Model file for the job. Use its own axes, mm. Give positions to 0.01 mm unless a question says otherwise; leave off trailing zeros. Loops run counter-clockwise (first coordinate to the right, second up) from the corner with the lowest first, then second, coordinate; pieces in that order, holes last. Notation, with made-up numbers: M -33.75,62 L 25.25,62 A17 cw 25.25,87 Z; hole C 69,12.5 d11. An arc over 180 degrees is marked long. Use CSV: the item, a comma, the result in double quotes. Start each with the question number.
(1) Wall check: line 1 along Y through (x, z) = (-37.05, 0.45); line 2 along Y through (x, z) = (-31.5, -0.8) (3 decimals); line 3 along Y through (x, z) = (27.05, -0.65). Give the ranges that are in metal, low to high. Write a range as from..to.
(2) Slice it at B-B on x = 27.05. List the corners of the cut face in (y, z).
(3) Slice it at C-C on y = -4.5. List the corners of the cut face in (x, z), and give its area (3 significant figures).
(4) Slice it at A-A on y = 12. List the corners of the cut face in (x, z) (3 decimals).
(5) Slice it at D-D on y = -19.5. List the corners of the cut face in (x, z).
(6) Flat gauge pins, fed straight in: P1, Ø0.9, axis at x = -25, z = -0.5, coming from the +Y side; P2, Ø4, axis at x = 31.5, y = 12, coming from the +Z side. Where does each tip first touch, or does it go through?
```python
from build123d import *

# Parameters (mm, degrees)
SKETCH_1_W                  = 93
SKETCH_1_H                  = 51
EXTRUDE_1_DEPTH             = 1.5
SKETCH_2_R                  = 1.525
CUT_EXTRUDE_1_DEPTH         = 5
HOLE_WIZARD_M3_1_AT_2_COUNT = 2
HOLE_WIZARD_M3_1_AT_2_PITCH = 63
SKETCH_5_R                  = 1.5
CUT_EXTRUDE_2_DEPTH         = 5
SKETCH_7_W                  = 20
SKETCH_7_H                  = 24
CUT_EXTRUDE_3_DEPTH         = 10
FILLET_1_R                  = 2
SKETCH_8_W                  = 16.1
SKETCH_8_H                  = 3.1
CUT_EXTRUDE_4_DEPTH         = 3
MIRROR_5_COPY_1_SKETCH_W    = 16.1
MIRROR_5_COPY_1_SKETCH_H    = 3.1
MIRROR_5_COPY_1_DEPTH       = 3
SKETCH_9_R                  = 1.025
CUT_EXTRUDE_5_DEPTH         = 3


with BuildPart() as part:
    # 草图1 → 凸台-拉伸1 (new body, symmetric)
    with BuildSketch(Plane.XY):
        Rectangle(SKETCH_1_W, SKETCH_1_H)
    extrude(amount=EXTRUDE_1_DEPTH, both=True)

    # 草图2 → 切除-拉伸1 (cut, symmetric)
    with BuildSketch(Plane.XY.offset(1.5)):
        with Locations((-31.5, 12)):
            Circle(SKETCH_2_R)
        with Locations((31.5, 12)):
            Circle(SKETCH_2_R)
    cut_extrude_1 = extrude(amount=CUT_EXTRUDE_1_DEPTH, both=True, mode=Mode.SUBTRACT)

    # 草图4 → M3 十字槽半沉头木螺钉的锥形沉头孔1 (revolve, cut)
    with BuildSketch(Plane(origin=(-31.5, 12, 1.5), x_dir=(0, -1, 0), z_dir=(1, 0, 0))):
        Polygon((0, 0), (0, 12.401290929), (1.5, 11.5), (1.5, 1.8), (3.3, 0), align=None)
    hole_wizard_m3_1 = revolve(axis=Axis((-31.5, 12, 7.85), (0, 0, -1)), mode=Mode.SUBTRACT)

    # M3 十字槽半沉头木螺钉的锥形沉头孔1 at 2: M3 十字槽半沉头木螺钉的锥形沉头孔1 ×2
    with Locations(*[(i * HOLE_WIZARD_M3_1_AT_2_PITCH, 0, 0) for i in range(1, HOLE_WIZARD_M3_1_AT_2_COUNT)]):
        add(hole_wizard_m3_1, mode=Mode.SUBTRACT)

    # 草图5 → 切除-拉伸2 (cut, symmetric)
    with BuildSketch(Plane(origin=(0, 0, -1.5), x_dir=(-1, 0, 0), z_dir=(0, 0, -1))):
        with Locations((-27.05, 4.5)):
            Circle(SKETCH_5_R)
        with Locations((-37.05, 4.5)):
            Circle(SKETCH_5_R)
        with Locations((-37.05, 19.5)):
            Circle(SKETCH_5_R)
        with Locations((-27.05, 19.5)):
            Circle(SKETCH_5_R)
        with Locations((27.05, 19.5)):
            Circle(SKETCH_5_R)
        with Locations((37.05, 19.5)):
            Circle(SKETCH_5_R)
        with Locations((37.05, 4.5)):
            Circle(SKETCH_5_R)
        with Locations((27.05, 4.5)):
            Circle(SKETCH_5_R)
    cut_extrude_2 = extrude(amount=CUT_EXTRUDE_2_DEPTH, both=True, mode=Mode.SUBTRACT)

    # 镜向1: 切除-拉伸2 across plane
    add(cut_extrude_2.mirror(Plane.ZX), mode=Mode.SUBTRACT)

    # 镜向2: M3 十字槽半沉头木螺钉的锥形沉头孔1, 切除-拉伸1 across plane
    add(hole_wizard_m3_1.mirror(Plane.ZX), mode=Mode.SUBTRACT)
    add(cut_extrude_1.mirror(Plane.ZX), mode=Mode.SUBTRACT)

    # 镜向2 copy 1 sketch → 镜向2 copy 1 (revolve, cut)
    with BuildSketch(Plane(origin=(31.5, -12, 1.5), x_dir=(0, 1, 0), z_dir=(1, 0, 0))):
        Polygon((0, 0), (0, -12.401290929), (1.5, -11.5), (1.5, -1.8), (3.3, 0), align=None)
    revolve(axis=Axis((31.5, -12, 7.85), (0, 0, 1)), mode=Mode.SUBTRACT)

    # 草图7 → 切除-拉伸3 (cut)
    with BuildSketch(Plane(origin=(0, 0, -1.5), x_dir=(-1, 0, 0), z_dir=(0, 0, -1))):
        with Locations((0, -25.5)):
            Rectangle(SKETCH_7_W, SKETCH_7_H)
    cut_extrude_3 = extrude(amount=-CUT_EXTRUDE_3_DEPTH, mode=Mode.SUBTRACT)

    # 镜向3: 切除-拉伸3 across plane
    add(cut_extrude_3.mirror(Plane.ZX), mode=Mode.SUBTRACT)

    # 圆角1
    fillet_1_edges = [part.edges().sort_by_distance(p)[0] for p in [
        (-10, -25.5, 0),
        (-10, -13.5, 0),
        (10, -25.5, 0),
        (10, -13.5, 0),
        (-10, 13.5, 0),
        (10, 13.5, 0),
        (-10, 25.5, 0),
        (10, 25.5, 0),
        (46.5, -25.5, 0),
        (-46.5, -25.5, 0),
        (-46.5, 25.5, 0),
        (46.5, 25.5, 0),
    ]]
    fillet(fillet_1_edges, radius=FILLET_1_R)

    # 草图8 → 切除-拉伸4 (cut)
    with BuildSketch(Plane(origin=(0, 0, -1.5), x_dir=(-1, 0, 0), z_dir=(0, 0, -1))):
        with Locations((-24.5, 24)):
            Rectangle(SKETCH_8_W, SKETCH_8_H)
    cut_extrude_4 = extrude(amount=-CUT_EXTRUDE_4_DEPTH, mode=Mode.SUBTRACT)

    # 镜向4: 切除-拉伸4 across plane
    add(cut_extrude_4.mirror(Plane(origin=(0, 0, 0), x_dir=(0, 0, 1), z_dir=(1, 0, 0))), mode=Mode.SUBTRACT)

    # 镜向5: 切除-拉伸4 across plane
    add(cut_extrude_4.mirror(Plane.ZX), mode=Mode.SUBTRACT)

    # 镜向5 copy 1 sketch → 镜向5 copy 1 (cut)
    with BuildSketch(Plane(origin=(0, 0, -1.5), x_dir=(1, 0, 0), z_dir=(0, 0, -1))):
        with Locations((-24.5, 24)):
            Rectangle(MIRROR_5_COPY_1_SKETCH_W, MIRROR_5_COPY_1_SKETCH_H)
    extrude(amount=-MIRROR_5_COPY_1_DEPTH, mode=Mode.SUBTRACT)

    # 草图9 → 切除-拉伸5 (cut)
    with BuildSketch(Plane.XY.offset(1.5)):
        with Locations((-31.525, 22.45)):
            Circle(SKETCH_9_R)
        with Locations((-17.475, 22.45)):
            Circle(SKETCH_9_R)
        with Locations((17.475, 22.45)):
            Circle(SKETCH_9_R)
        with Locations((31.525, 22.45)):
            Circle(SKETCH_9_R)
    cut_extrude_5 = extrude(amount=-CUT_EXTRUDE_5_DEPTH, mode=Mode.SUBTRACT)

    # 镜向6: 切除-拉伸5 across plane
    add(cut_extrude_5.mirror(Plane.ZX), mode=Mode.SUBTRACT)


solid = part.part
```
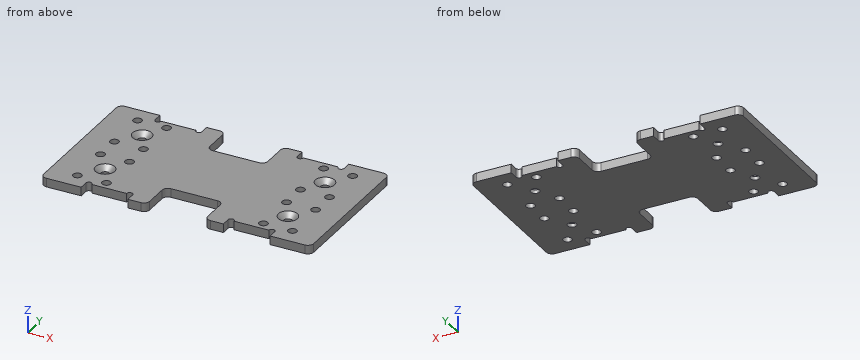
Reply:
1,line 1,"y = -25.5..-21, -18..-6, -3..3, 6..18, 21..25.5"
1,line 2,"y = -21.425..-13.525, -10.475..10.475, 13.525..21.425"
1,line 3,"y = -22.45..-21, -18..-6, -3..3, 6..18, 21..22.45"
2,outline,"M -22.45,-1.5 L -21,-1.5 L -21,1.5 L -22.45,1.5 Z; M -18,-1.5 L -6,-1.5 L -6,1.5 L -18,1.5 Z; M -3,-1.5 L 3,-1.5 L 3,1.5 L -3,1.5 Z; M 6,-1.5 L 18,-1.5 L 18,1.5 L 6,1.5 Z; M 21,-1.5 L 22.45,-1.5 L 22.45,1.5 L 21,1.5 Z"
3,outline,"M -46.5,-1.5 L -38.55,-1.5 L -38.55,1.5 L -46.5,1.5 Z; M -35.55,-1.5 L -28.55,-1.5 L -28.55,1.5 L -35.55,1.5 Z; M -25.55,-1.5 L 25.55,-1.5 L 25.55,1.5 L -25.55,1.5 Z; M 28.55,-1.5 L 35.55,-1.5 L 35.55,1.5 L 28.55,1.5 Z; M 38.55,-1.5 L 46.5,-1.5 L 46.5,1.5 L 38.55,1.5 Z"
3,area,"243 mm^2"
4,outline,"M -46.5,-1.5 L -33.025,-1.5 L -33.025,-0.275 L -34.8,1.5 L -46.5,1.5 Z; M -29.975,-1.5 L 29.975,-1.5 L 29.975,-0.275 L 28.2,1.5 L -28.2,1.5 L -29.975,-0.275 Z; M 33.025,-1.5 L 46.5,-1.5 L 46.5,1.5 L 34.8,1.5 L 33.025,-0.275 Z"
5,outline,"M -46.5,-1.5 L -38.55,-1.5 L -38.55,1.5 L -46.5,1.5 Z; M -35.55,-1.5 L -28.55,-1.5 L -28.55,1.5 L -35.55,1.5 Z; M -25.55,-1.5 L -10,-1.5 L -10,1.5 L -25.55,1.5 Z; M 10,-1.5 L 25.55,-1.5 L 25.55,1.5 L 10,1.5 Z; M 28.55,-1.5 L 35.55,-1.5 L 35.55,1.5 L 28.55,1.5 Z; M 38.55,-1.5 L 46.5,-1.5 L 46.5,1.5 L 38.55,1.5 Z"
6,P1,"stops at y = 22.45"
6,P2,"stops at z = 0.2"
